from build123d import *

# Parameters (mm, degrees)
BOSS_EXTRUDE3_DEPTH  = 10
SKETCH1_6_W          = 12
SKETCH1_6_H          = 40
BOSS_EXTRUDE4_DEPTH  = 80
FILLET1_R            = 20
BOSS_EXTRUDE5_DEPTH  = 40
BOSS_EXTRUDE11_DEPTH = 5
SKETCH12_R           = 5
CUT_EXTRUDE1_DEPTH   = 148.732867027


with BuildPart() as part:
    # Sketch1 → Boss-Extrude3 (new body)
    with BuildSketch(Plane(origin=(0, 0, 0), x_dir=(1, 0, 0), z_dir=(0, 1, 0))):
        with BuildLine():
            Line((57, -40), (12, -40))
            Line((12, -40), (12, -80))
            ThreePointArc((12, -80), (17.481881586, -72.752551286), (26.142135624, -70))
            Line((26.142135624, -70), (77, -70))
            Line((77, -70), (77, -60))
            ThreePointArc((77, -60), (62.857864376, -54.142135624), (57, -40))
        make_face()
        with BuildLine():
            ThreePointArc((26.142135624, -10), (17.481881586, -7.247448714), (12, 0))
            Line((12, 0), (12, -40))
            Line((12, -40), (57, -40))
            ThreePointArc((57, -40), (62.857864376, -25.857864376), (77, -20))
            Line((77, -20), (77, -10))
            Line((77, -10), (26.142135624, -10))
        make_face()
        with BuildLine():
            ThreePointArc((107, -40), (98.213203436, -18.786796564), (77, -10))
            Line((77, -10), (77, -20))
            ThreePointArc((77, -20), (91.142135624, -25.857864376), (97, -40))
            Line((97, -40), (107, -40))
        make_face()
        with BuildLine():
            ThreePointArc((97, -40), (91.142135624, -54.142135624), (77, -60))
            Line((77, -60), (77, -70))
            ThreePointArc((77, -70), (98.213203436, -61.213203436), (107, -40))
            Line((107, -40), (97, -40))
        make_face()
    extrude(amount=BOSS_EXTRUDE3_DEPTH)

    # Sketch1_6 → Boss-Extrude4 (add)
    with BuildSketch(Plane(origin=(0, 0, 0), x_dir=(1, 0, 0), z_dir=(0, 1, 0))):
        with Locations((6, -20)):
            Rectangle(SKETCH1_6_W, SKETCH1_6_H)
        with Locations((6, -60)):
            Rectangle(SKETCH1_6_W, SKETCH1_6_H)
    extrude(amount=BOSS_EXTRUDE4_DEPTH)

    # Fillet1
    fillet1_edges = [part.edges().sort_by_distance(p)[0] for p in [
        (6, 80, 80),
        (6, 80, 0),
    ]]
    fillet(fillet1_edges, radius=FILLET1_R)

    # Sketch1_8 → Boss-Extrude5 (add)
    with BuildSketch(Plane(origin=(0, 0, 0), x_dir=(1, 0, 0), z_dir=(0, 1, 0))):
        with BuildLine():
            ThreePointArc((77, -20), (62.857864376, -25.857864376), (57, -40))
            Line((57, -40), (64.5, -40))
            ThreePointArc((64.5, -40), (68.161165235, -31.161165235), (77, -27.5))
            Line((77, -27.5), (77, -20))
        make_face()
        with BuildLine():
            Line((64.5, -40), (57, -40))
            ThreePointArc((57, -40), (62.857864376, -54.142135624), (77, -60))
            Line((77, -60), (77, -52.5))
            ThreePointArc((77, -52.5), (68.161165235, -48.838834765), (64.5, -40))
        make_face()
        with BuildLine():
            ThreePointArc((97, -40), (91.142135624, -25.857864376), (77, -20))
            Line((77, -20), (77, -27.5))
            ThreePointArc((77, -27.5), (85.838834765, -31.161165235), (89.5, -40))
            Line((89.5, -40), (97, -40))
        make_face()
        with BuildLine():
            Line((77, -52.5), (77, -60))
            ThreePointArc((77, -60), (91.142135624, -54.142135624), (97, -40))
            Line((97, -40), (89.5, -40))
            ThreePointArc((89.5, -40), (85.838834765, -48.838834765), (77, -52.5))
        make_face()
    extrude(amount=BOSS_EXTRUDE5_DEPTH)

    # Sketch11 → Boss-Extrude11 (add, symmetric)
    with BuildSketch(Plane.XY.offset(40)):
        with BuildLine():
            Line((12, 80), (12, 10))
            Line((12, 10), (57, 10))
            Line((57, 10), (64.5, 10))
            Line((64.5, 10), (64.5, 40))
            Line((64.5, 40), (57, 40))
            ThreePointArc((57, 40), (27.804407401, 52.467458326), (12, 80))
        make_face()
    extrude(amount=BOSS_EXTRUDE11_DEPTH, both=True)

    # Sketch12 → Cut-Extrude1 (cut, through all)
    with BuildSketch(Plane(origin=(12, 0, 0), x_dir=(0, 0, -1), z_dir=(1, 0, 0))):
        with Locations((-65, 60)):
            Circle(SKETCH12_R)
        with Locations((-15, 60)):
            Circle(SKETCH12_R)
    extrude(amount=-CUT_EXTRUDE1_DEPTH, mode=Mode.SUBTRACT)


solid = part.part
The listing builds one solid part. Answer for the finished solid, in the listing's coordinates (mm). A direction names the side the tool comes from. Round coordinates to 2 decimals unless told otherwise and drop trailing zeros. Order: outer loops, then holes, each group sorted by start corner. A loop starts at its lowest first (then second) coordinate and runs counter-clockwise, first axis right, second up. Notation, with made-up numbers: (71, 65.25) - (78, 65.25) arc R19 ccw to (78, 99.25) - close; hole circle Ø6 at (44.5, -24.75). An arc over 180 degrees is marked (long way). Write item = value, one per line. Start each with the question number.
1) Section C-C, the plane z = 63 is taken. Write down the section's boundary in (x, y), plus the area to 3 significant figures.
2) Given pin 1 (5 mm diameter, centred on y = 61, z = 46.5, fed in from +X) (3 decimals); pin 2 (5 mm diameter, centred on x = 21.5, y = 53.5, fed in from -Z); pin 3 (3 mm diameter, centred on x = 27, z = 18, fed in from +Y), each flat-ended and moving along its own axis, determine where each tip first touches the part or whether it passes through.
3) For faces 1 (the flat face through (48, 10, 48)), 2 (the flat face through (52, 5, 10)), 3 (the flat face through (29, 30, 45)), 4 (the flat face through (51, 5, 70)), 5 (the flat face through (12, 45, 18)), determine the directions among +Z, -Z, +X, -X, +Y, -Y from which every point of the face is accessible in a straight line to the end or side of a thin tool.
4) Section D-D, the plane x = 43.5 is taken. Write down the section's boundary in (y, z).
5) For a pull along X with two mould halves and no side action, classify faces 6 (the cylindrical face through (17.377, 4.93, 72.828)), 7 (the flat face through (29, 30, 35)), 8 (the flat face through (86, 40, 31)) as released by +X, released by -X, zero draft, split by the parting line, or undercut.
6) Section A-A, the plane x = 85 is taken. Write down the section's boundary in (y, z).
7) Straight lines are drawn through the part: L1, parallel to X at y = 37, z = 45.5; L2, parallel to X at y = 49, z = 27.5; L3, parallel to Y at x = 56.5, z = 64. For each, find the intervals that lie inside material, in ascending order.
8) Section B-B, the plane y = 57 is taken. Write down the section's boundary in (x, z).
Results list:
q1.outline = (0, 0) - (96.26, 0) - (96.26, 10) - (12, 10) - (12, 55.42) - (0, 55.42) - close; (0, 64.58) - (12, 64.58) - (12, 79.77) - (0, 79.77) - close
q1.area = 1,690 mm^2
q2.pin_1 = 21.665
q2.pin_2 = 35
q2.pin_3 = 10
q3.face_1 = +Y
q3.face_2 = -Z, +X, +Y, -Y
q3.face_3 = +Z, +Y
q3.face_4 = +Z, +X, +Y, -Y
q3.face_5 = -Z, +Y
q4.outline = (0, 10) - (10, 10) - (10, 35) - (43.01, 35) - (43.01, 45) - (10, 45) - (10, 70) - (0, 70) - close
q5.face_6 = released by +X
q5.face_7 = undercut
q5.face_8 = zero draft
q6.outline = (0, 11.09) - (10, 11.09) - (10, 21.67) - (40, 21.67) - (40, 30.4) - (0, 30.4) - close; (0, 49.6) - (40, 49.6) - (40, 58.33) - (10, 58.33) - (10, 68.91) - (0, 68.91) - close
q7.L1 = 0 to 12, 57.77 to 65.78, 88.22 to 96.23
q7.L2 = 0 to 12
q7.L3 = 0 to 10
q8.outline = (0, 0) - (12, 0) - (12, 11) - (0, 11) - close; (0, 19) - (12, 19) - (12, 35) - (23.32, 35) - (23.32, 45) - (12, 45) - (12, 61) - (0, 61) - close; (0, 69) - (12, 69) - (12, 80) - (0, 80) - close
